Autodesk Inventor part; units mm, degrees
ref_plane "YZ Plane" through (0, 0, 0) normal (1, 0, 0) x (0, 1, 0)
ref_plane "XZ Plane" through (0, 0, 0) normal (0, 1, 0) x (-1, 0, 0)
ref_plane "XY Plane" through (0, 0, 0) normal (0, 0, 1) x (1, 0, 0)
sketch "スケッチ1" plane through (0, 0, 0) normal (0, 1, 0) x (-1, 0, 0)
  line L0 (0, 0) -> (6, 0)
  line L1 (6, 0) -> (6, -3)
  line L2 (6, -3) -> (0, -3)
  line L3 (0, -3) -> (0, 0)
  dimension "d0" = 6
  dimension "d1" = 3
revolve "回転1" add sketch "スケッチ1" angle 360 about axis through (0, 0, 0) along (-1, 0, 0)
sketch "スケッチ2" plane through (0, 0, 0) normal (1, 0, 0) x (0, 0, -1)
  point P0 (0, 0)
  point P1 (0, 0)
hole "穴1" at (0, 0, 0) direction (-1, 0, 0) diameter 2.459 end through all
sketch "スケッチ3" plane through (0, 0, 0) normal (1, 0, 0) x (0, 0, -1)
  circle A0 centre (0, 0) radius 3
  line L0 (3, 0) -> (-3, 0)
  line L1 (3, -0.5) -> (-3, -0.5)
  line L2 (3, 0.5) -> (-3, 0.5)
  line L3 (3, 0.5) -> (3, -0.5)
  line L4 (-3, 0.5) -> (-3, -0.5)
  point P0 (-2.958, -0.5)
  point P1 (2.958, -0.5)
  point P2 (2.958, 0.5)
  point P3 (-2.958, 0.5)
  dimension "d10" = 0.5
extrude "押し出し1" cut sketch "スケッチ3" against normal blind 1 contours L0 A0 L2 | A0 L1 L0
chamfer "面取り1" distance 0.3 angle 45 3 edges at (-6, 0, 3) (0, 3, 0) (0, -3, 0)
properties part number "ARU-306S" material "ステンレス鋼 AISI 304"
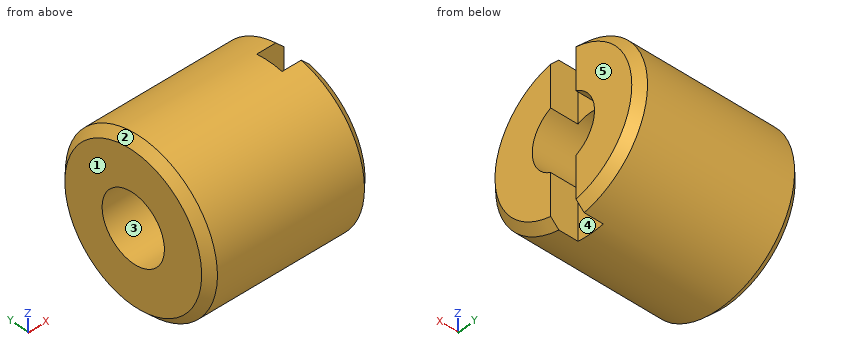
Verification items for the finished model (mm, model axes). Face numbers are marked on the shaded views. A direction names the side the tool comes from. Give positions to 0.01 mm unless a question says otherwise; leave off trailing zeros. Write each loop counter-clockwise with the first axis right and the second up, starting at its lowest first coordinate (ties: lowest second). Pieces come first, ordered by that corner, then holes. Notation, with made-up numbers: M 28.25,53 L 53.25,53 A27 ccw 53.25,81 Z; hole C 13.25,34.5 d6. An arc over 180 degrees is marked long. Put each result on its own line as item: value. Start each with the question number.
1. Set-up check for the marked faces 4 and 5: record each of +Z, -Z, +X, -X, +Y, -Y from which the full face is reachable in a straight line by a thin tool's end or side.
2. Go/stop test with flat-tipped pins: pin 1 Ø1.1 at (x, z) = (-0.5, 2) entering from +Y; pin 2 Ø1.5 at (x, z) = (-4.5, -2.5) entering from +Y; pin 3 Ø0.8 at (y, z) = (0, 2) entering from +X. Record where each tip stops, or that it passes through.
3. Scan lines: line 1 along Z through (x, y) = (-3.9, 0); line 2 along Y through (x, z) = (-1.05, 0.5). Record each from-to range of solid material in increasing order. Write a range as [from, to].
4. Section check A-A (z = 0). Record the cut outline in (x, y).
5. Section check C-C (x = -2.2). Record the cut outline in (y, z), and give its area (3 significant figures).
6. Draft check along Z on the marked faces 1, 2 and 3. Enter one of: +Z half, -Z half, draft (parallel to the pull), parting line (faces both ways), or undercut.
7. Section check B-B (y = 0). Record the cut outline in (x, z), and give its area (3 significant figures).
Answer list:
1. face 4: +Z, -Z, +X
1. face 5: +Z, -Z, +X, +Y, -Y
2. pin 1: y = 2.63
2. pin 2: y = 2.44
2. pin 3: x = -1
3. line 1: [-3, -1.23], [1.23, 3]
3. line 2: [-2.96, -1.12], [1.12, 2.96]
4. outline: M -6,-2.7 L -5.7,-3 L -0.3,-3 L 0,-2.7 L 0,-1.23 L -6,-1.23 Z; M -6,1.23 L 0,1.23 L 0,2.7 L -0.3,3 L -5.7,3 L -6,2.7 Z
5. outline: C 0,0 d6; hole C 0,0 d2.46
5. area: 23.5 mm2
6. face 1: draft
6. face 2: parting line
6. face 3: undercut
7. outline: M -6,-2.7 L -5.7,-3 L -1,-3 L -1,-1.23 L -6,-1.23 Z; M -6,1.23 L -1,1.23 L -1,3 L -5.7,3 L -6,2.7 Z
7. area: 17.6 mm2
